For this review, take the finished solid that the model builds, in its own axes (mm). A direction names the side the tool comes from. Give positions to 0.01 mm unless a question says otherwise; leave off trailing zeros. Order: outer loops, then holes, each group sorted by start corner. A loop starts at its lowest first (then second) coordinate and runs counter-clockwise, first axis right, second up. Notation, with made-up numbers: (64, 78.5) - (79, 78.5) arc R23 ccw to (79, 113.5) - close; hole circle Ø10 at (22.25, 29). An arc over 180 degrees is marked (long way). One line per item, written item: value.
```python
from build123d import *

# Parameters (mm, degrees)
SKETCH1_R           = 8
BOSS_EXTRUDE2_DEPTH = 2
SKETCH2_W           = 0.5
SKETCH2_H           = 0.6


with BuildPart() as part:
    # Sketch1 → Boss-Extrude2 (new body)
    with BuildSketch(Plane.XY):
        Circle(SKETCH1_R)
        with BuildLine():
            Line((-1.549193338, -1.1), (1.549193338, -1.1))
            ThreePointArc((1.549193338, -1.1), (0, 1.9), (-1.549193338, -1.1))
        make_face(mode=Mode.SUBTRACT)
    extrude(amount=BOSS_EXTRUDE2_DEPTH)

    # Sketch2 → Cut-Revolve1 (revolve, cut)
    with BuildSketch(Plane(origin=(0, 0, 0), x_dir=(1, 0, 0), z_dir=(0, 1, 0)), mode=Mode.PRIVATE) as cut_revolve1_sk:
        with Locations((-7.75, -1)):
            Rectangle(SKETCH2_W, SKETCH2_H)
    revolve(cut_revolve1_sk.sketch.rotate(Axis((0, 0, 2), (0, 0, -1)), 180), axis=Axis((0, 0, 2), (0, 0, -1)), mode=Mode.SUBTRACT)


solid = part.part
```
(1) Take a section at A-A (x = 0). Write out the cut boundary in (y, z), then the cut area to 3 significant figures.
Answers below:
outline: (-8, 0) - (-1.1, 0) - (-1.1, 2) - (-8, 2) - (-8, 1.3) - (-7.5, 1.3) - (-7.5, 0.7) - (-8, 0.7) - close; (1.9, 0) - (8, 0) - (8, 0.7) - (7.5, 0.7) - (7.5, 1.3) - (8, 1.3) - (8, 2) - (1.9, 2) - close
area: 25.4 mm^2
(2) Wall thickness on line 1 (Y direction, x = 0, z = 1.1); line 2 (X direction, y = 0, z = 0.55); line 3 (Y direction, x = 0, z = 0.5): over which ranges is each line inside the solid? List them lowest first. Write a range as from..to.
Answers below:
line 1: y = -7.5..-1.1, 1.9..7.5
line 2: x = -8..-1.9, 1.9..8
line 3: y = -8..-1.1, 1.9..8
(3) Take a section at D-D (y = 6.75). Write out the cut boundary in (x, z), then the cut area to 3 significant figures.
Answers below:
outline: (-4.29, 0) - (4.29, 0) - (4.29, 0.7) - (3.27, 0.7) - (3.27, 1.3) - (4.29, 1.3) - (4.29, 2) - (-4.29, 2) - (-4.29, 1.3) - (-3.27, 1.3) - (-3.27, 0.7) - (-4.29, 0.7) - close
area: 15.9 mm^2
(4) Take a section at B-B (y = 0). Write out the cut boundary in (x, z), then the cut area to 3 significant figures.
Answers below:
outline: (-8, 0) - (-1.9, 0) - (-1.9, 2) - (-8, 2) - (-8, 1.3) - (-7.5, 1.3) - (-7.5, 0.7) - (-8, 0.7) - close; (1.9, 0) - (8, 0) - (8, 0.7) - (7.5, 0.7) - (7.5, 1.3) - (8, 1.3) - (8, 2) - (1.9, 2) - close
area: 23.8 mm^2
(5) For P1, Ø1, axis at x = 0, z = 1, coming from the +Y side, flat-tipped, find the tip position at first contact; note if it passes through.
Answers below:
P1: stops at y = 8
(6) Machinability: for faces 1 (the face through (0, -2, 2)), 2 (the face through (5, 6, 1.3)), which of the approach directions +Z, -Z, +X, -X, +Y, -Y give a long, thin tool a straight path to every point of the face, cutting with its end or side? Answer none if there is none.
Answers below:
face 1: +Z, +X, -X, +Y, -Y
face 2: none
(7) Draft analysis for pull direction Y (two halves, no side actions). For faces 3 (the face through (0, -1.1, 1)), 4 (the face through (0.06, 1.9, 0.99)), 5 (the face through (0, -2, 0)), 6 (the face through (-1.73, -7.81, 0.35)), state which applies: pulls with the +Y half, pulls with the -Y half, needs draft (parallel to the pull), parting line crosses it, or undercut.
Answers below:
face 3: undercut
face 4: undercut
face 5: needs draft
face 6: parting line crosses it
(8) Take a section at C-C (z = 1.5). Write out the cut boundary in (x, y), then the cut area to 3 significant figures.
Answers below:
outline: circle Ø16 at (0, 0); hole (-1.55, -1.1) - (1.55, -1.1) arc R1.9 ccw (long way) to start
area: 191 mm^2
